from build123d import *

# Parameters (mm, degrees)
BOSS_EXTRUDE1_DEPTH             = 3.2
SKETCH2_R                       = 2.5
CUT_EXTRUDE1_DEPTH              = 1601.073510811
F_4_0MM_DOWEL_HOLE1_D           = 4
F_4_0MM_DOWEL_HOLE1_CSINK_D     = 4.05
F_4_0MM_DOWEL_HOLE1_CSINK_ANGLE = 90
LPATTERN2_COUNT                 = 30
LPATTERN2_PITCH                 = 54


with BuildPart() as part:
    # Sketch1 → Boss-Extrude1 (new body)
    with BuildSketch(Plane(origin=(0, 0, 0), x_dir=(1, 0, 0), z_dir=(0, 1, 0))):
        with BuildLine():
            Line((0, 12), (0, 0))
            Line((0, 0), (15, 0))
            Line((15, 0), (15, 12))
            ThreePointArc((15, 12), (13.232233047, 12.732233047), (12.5, 14.5))
            Line((12.5, 14.5), (12.5, 1585.5))
            ThreePointArc((12.5, 1585.5), (13.232233047, 1587.267766953), (15, 1588))
            Line((15, 1588), (15, 1600))
            Line((15, 1600), (0, 1600))
            Line((0, 1600), (0, 1588))
            ThreePointArc((0, 1588), (1.767766953, 1587.267766953), (2.5, 1585.5))
            Line((2.5, 1585.5), (2.5, 14.5))
            ThreePointArc((2.5, 14.5), (1.767766953, 12.732233047), (0, 12))
        make_face()
    extrude(amount=BOSS_EXTRUDE1_DEPTH)

    # Sketch2 → Cut-Extrude1 (cut, through all)
    with BuildSketch(Plane(origin=(0, 3.2, 0), x_dir=(1, 0, 0), z_dir=(0, 1, 0))):
        with Locations(Location((7.5, 17, 0), (0, 0, 270))):
            Circle(SKETCH2_R)
    cut_extrude1 = extrude(amount=-CUT_EXTRUDE1_DEPTH, mode=Mode.SUBTRACT)

    # Ø4.0mm Dowel Hole1 (through all)
    with Locations(Plane(origin=(11.5, 3.2, -1591), x_dir=(0, 0, 1), z_dir=(0, 1, 0))):
        with Locations((0, 0), (0, -8), (-6, -8), (-6, 0), (1582, -8), (1588, -8), (1582, 0), (1588, 0)):
            CounterSinkHole(F_4_0MM_DOWEL_HOLE1_D / 2, F_4_0MM_DOWEL_HOLE1_CSINK_D / 2, counter_sink_angle=F_4_0MM_DOWEL_HOLE1_CSINK_ANGLE)

    # LPattern2: Cut-Extrude1 ×30
    with Locations(*[(0, 0, -i * LPATTERN2_PITCH) for i in range(1, LPATTERN2_COUNT)]):
        add(cut_extrude1, mode=Mode.SUBTRACT)


solid = part.part
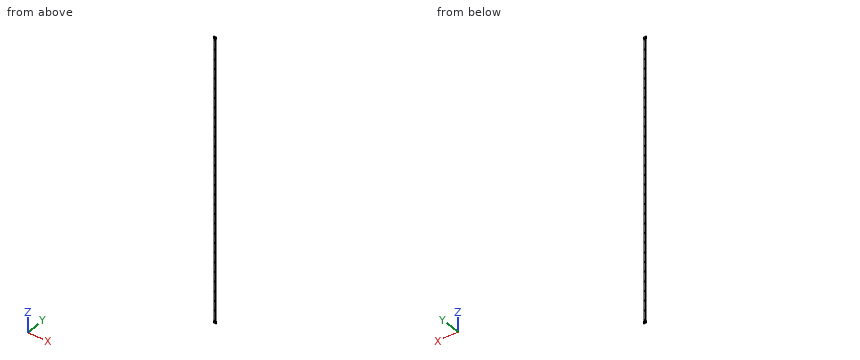
Part model, mm, in its own coordinate system. Give positions to 0.01 mm unless a question says otherwise; leave off trailing zeros. Loops run counter-clockwise (first coordinate to the right, second up) from the corner with the lowest first, then second, coordinate; pieces in that order, holes last. Notation, with made-up numbers: (-4.5, 72) -> (7.5, 72) arc R31 cw to (7.5, 109) -> close; hole circle Ø8 at (43.5, 19). An arc over 180 degrees is marked (long way). Write each question's results on one line, items separated by ' | '. Start each with the question number.
Q1. Wall check: L1, parallel to Z at x = 3.75, y = 1.3; L2, parallel to X at y = 2.5, z = -1591; L3, parallel to X at y = 1.45, z = -1205. Give the ranges that are in metal, low to high.
Q2. Pin check, flat tip, straight feed: P1, Ø2.5, axis at x = 3.5, z = -9, coming from the -Y side. Stop position of the tip, or through.
Q3. Band-saw the part on A-A on y = 0.65. Count the separate pieces of the cut face and the enclosed holes in it, plus the area to 3 significant figures.
Q4. Band-saw the part on B-B on z = -1067.5. List the corners of the cut face in (x, y), plus the area to 3 significant figures.
Results are:
1) L1: z = -1600 to -1598.98, -1595.02 to -1592.98, -1589.02 to -10.98, -7.02 to -4.98, -1.02 to 0 | L2: x = 0 to 1.5, 5.5 to 9.5, 13.5 to 15 | L3: x = 2.5 to 5, 10 to 12.5
2) P1: passes through
3) separate pieces: 1 | enclosed holes: 38 | area: 15,400 mm²
4) outline: (2.5, 0) -> (12.5, 0) -> (12.5, 3.2) -> (2.5, 3.2) -> close | area: 32.0 mm²
